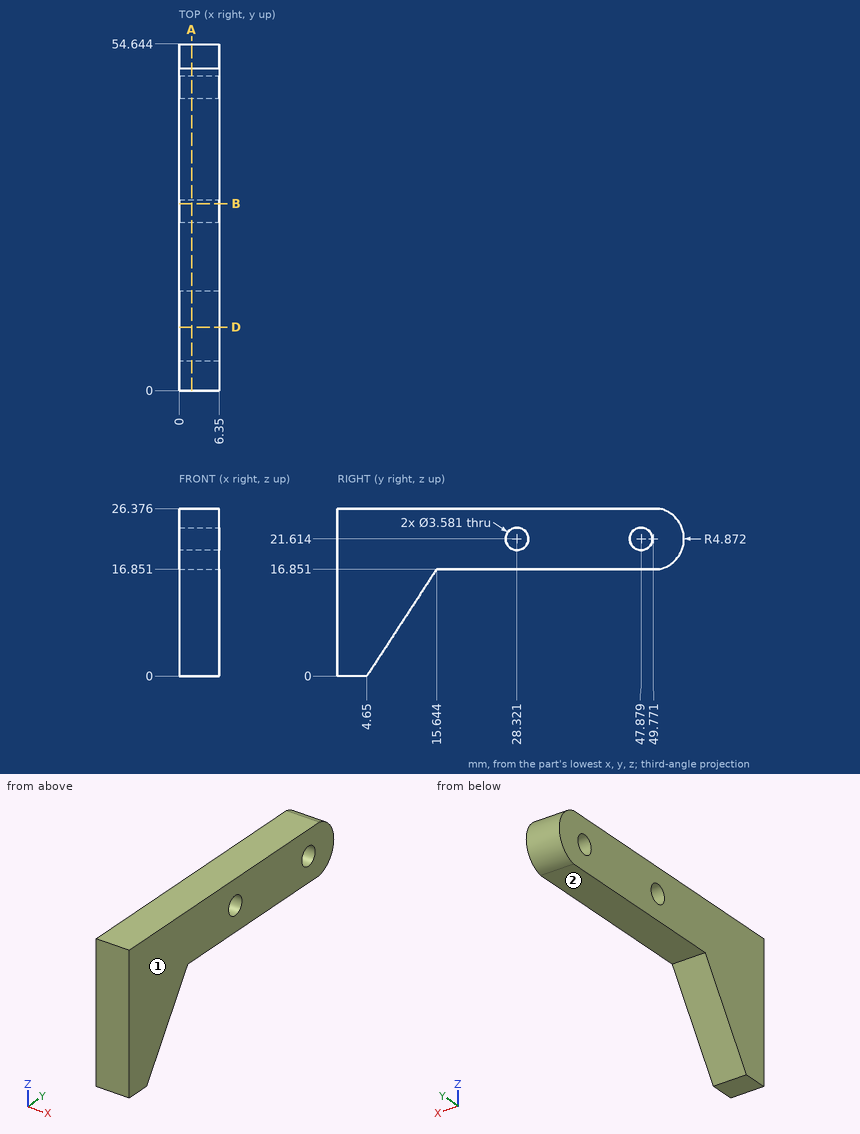
Check sheet for the drawn part. Datum: minimum x, y, z corner. Units: mm. A direction names the side the tool comes from. Give positions to 0.01 mm unless a question says otherwise; leave off trailing zeros. Loops run counter-clockwise (first coordinate to the right, second up) from the corner with the lowest first, then second, coordinate; pieces in that order, holes last.
1) Sectioned sample at A-A, the plane x = 2. Count the separate pieces of the cut face and the enclosed holes in it, then the cut area to 3 significant figures.
2) Sectioned sample at B-B, the plane y = 29.5. Enter the section's corners in (x, z).
3) Sectioned sample at D-D, the plane y = 10. Enter the section's corners in (x, z).
4) Depth check by flat-ended pin: pin 1 Ø4 at (y, z) = (47.88, 21.61) entering from +X; pin 2 Ø1.5 at (x, z) = (1, 19.5) entering from +Y; pin 3 Ø3 at (x, z) = (5, 5) entering from +Y. Enter the tip coordinate at first touch or a pass-through.
5) Thickness scan on line 1 along Z through (x, y) = (0.5, 46); line 2 along Y through (x, z) = (3, 20) (1 decimal); line 3 along Y through (x, z) = (5.75, 21.25) (1 decimal). Record the ranges inside material, lowest first.
6) Set-up check for the marked faces 1 and 2: record each of +Z, -Z, +X, -X, +Y, -Y from which the full face is reachable in a straight line by a thin tool's end or side.
Answers:
1. separate pieces: 1
1. enclosed holes: 2
1. area: 662 mm2
2. outline: (0, 16.85) - (6.35, 16.85) - (6.35, 20.27) - (0, 20.27) - close; (0, 22.96) - (6.35, 22.96) - (6.35, 26.38) - (0, 26.38) - close
3. outline: (0, 8.2) - (6.35, 8.2) - (6.35, 26.38) - (0, 26.38) - close
4. pin 1: stops at x = 6.35
4. pin 2: stops at y = 54.45
4. pin 3: stops at y = 8.89
5. line 1: z = 16.85 to 26.38
5. line 2: y = 0 to 27.5, 29.1 to 47.1, 48.7 to 54.4
5. line 3: y = 0 to 26.6, 30.1 to 46.1, 49.6 to 54.6
6. face 1: +Z, -Z, +X, +Y, -Y
6. face 2: -Z, +X, -X, +Y
